Job drawing, mm, ordinate dimensions from the low corner. One solid piece. A direction names the side the tool comes from. Give positions to 0.01 mm unless a question says otherwise; leave off trailing zeros. Loops run counter-clockwise (first coordinate to the right, second up) from the corner with the lowest first, then second, coordinate; pieces in that order, holes last. Notation, with made-up numbers: M 25.25,-27.5 L 61.25,-27.5 A18 ccw 61.25,-18.5 Z; hole C 60.5,-23.5 d8. An arc over 180 degrees is marked long. Answer as CSV lines item,"result".
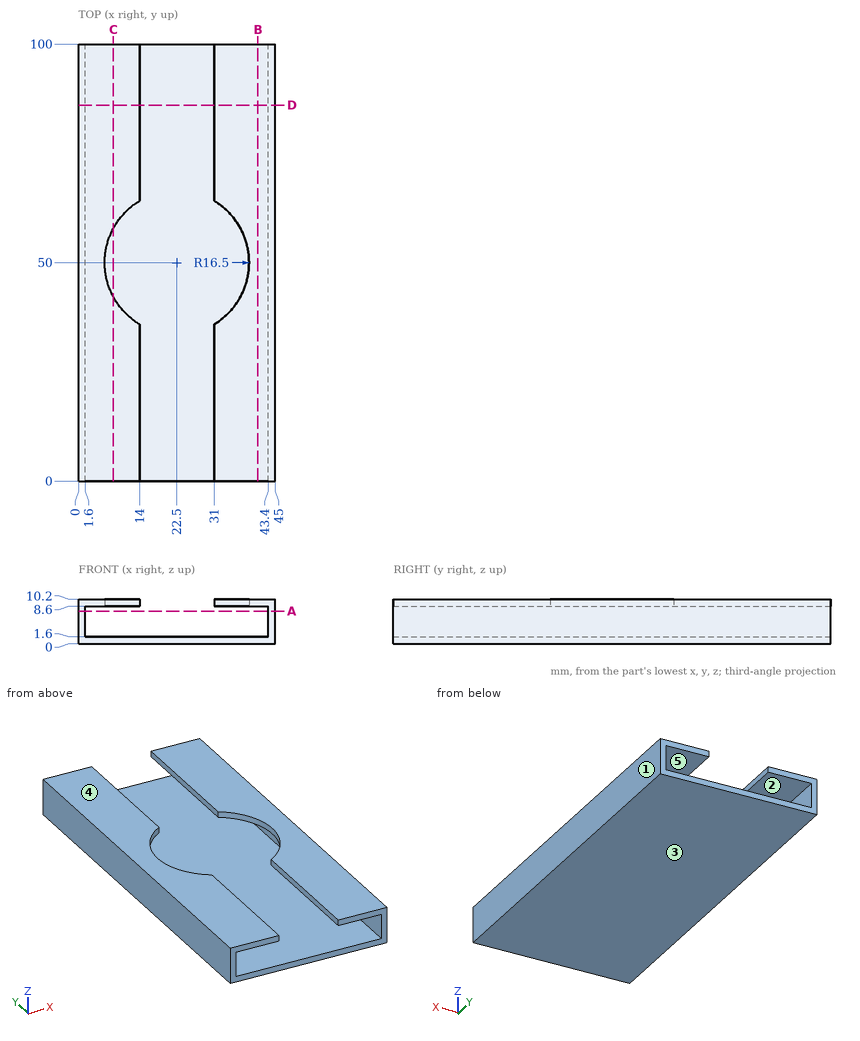
1) Which spindle directions (+Z, -Z, +X, -X, +Y, -Y) get a long thin tool onto all of the face, cutting with end or side? Do the marked faces 4 and 5. Say none if no direction does.
Answer below:
face 4,"+Z, +X, -X, +Y, -Y"
face 5,"+Y, -Y"
2) Flat gauge pin, fed straight in: pin 1 (1.5 mm diameter, centred on x = 12.5, y = 47.5, fed in from +Z). Where does the tip first touch, or does it go through?
Answer below:
pin 1,"stops at z = 1.6"
3) Band-saw the part on C-C on x = 8. Give the cut face in (y, z), and give its area (3 significant figures).
Answer below:
outline,"M 0,0 L 100,0 L 100,1.6 L 0,1.6 Z; M 0,8.6 L 42.13,8.6 L 42.13,10.2 L 0,10.2 Z; M 57.87,8.6 L 100,8.6 L 100,10.2 L 57.87,10.2 Z"
area,"295 mm^2"
4) Band-saw the part on D-D on y = 86. Give the cut face in (x, z).
Answer below:
outline,"M 0,0 L 45,0 L 45,10.2 L 31,10.2 L 31,8.6 L 43.4,8.6 L 43.4,1.6 L 1.6,1.6 L 1.6,8.6 L 14,8.6 L 14,10.2 L 0,10.2 Z"
5) Mould opens along X. For the marked faces 1, 2 and 3 say: +X half, -X half, draft (parallel to the pull), parting line (faces both ways), or undercut.
Answer below:
face 1,"+X half"
face 2,"undercut"
face 3,"draft"
6) Band-saw the part on B-B on x = 41. Give the cut face in (y, z), and give its area (3 significant figures).
Answer below:
outline,"M 0,0 L 100,0 L 100,1.6 L 0,1.6 Z; M 0,8.6 L 100,8.6 L 100,10.2 L 0,10.2 Z"
area,"320 mm^2"
7) Band-saw the part on A-A on z = 7.5. Give the cut face in (x, y), and give its area (3 significant figures).
Answer below:
outline,"M 0,0 L 1.6,0 L 1.6,100 L 0,100 Z; M 43.4,0 L 45,0 L 45,100 L 43.4,100 Z"
area,"320 mm^2"
8) Drill centre lines: line 1 (X direction, y = 74, z = 8.75); line 2 (X direction, y = 24.5, z = 8); line 3 (Z direction, x = 32, y = 18). Where is each one in solid material? Low to high. Write a range as from..to.
Answer below:
line 1,"x = 0..14, 31..45"
line 2,"x = 0..1.6, 43.4..45"
line 3,"z = 0..1.6, 8.6..10.2"
